Read the model definition and answer for the solid it produces. Units are mm, in the model's axes. Face numbers are marked on the shaded views. A direction names the side the tool comes from. Round coordinates to 2 decimals unless told otherwise and drop trailing zeros. Order: outer loops, then holes, each group sorted by start corner. A loop starts at its lowest first (then second) coordinate and runs counter-clockwise, first axis right, second up. Notation, with made-up numbers: (88, 85) - (140, 85) arc R21 cw to (140, 97) - close; hole circle Ø8 at (25.25, 75). An arc over 180 degrees is marked (long way). Answer as a JSON object with one key per item and string values. Group by question number.
Q1. A tool of negligible diameter and unlimited length cuts with its end or side. For the marked faces 1, 2 and 3, from which of +Z, -Z, +X, -X, +Y, -Y can it reach the whole face along a straight path? Write none if from no direction.
Q2. The mould has two halves that part along Y. Classify the marked faces 4, 5 and 6: pulls with the +Y half, pulls with the -Y half, needs draft (parallel to the pull), parting line crosses it, or undercut.
Q3. A cutting plane is placed at B-B on x = -11.5. Determine the outline of the cut face in (y, z).
Q4. Given pin 1 Ø2 at (x, y) = (14.5, -5) entering from -Z; pin 2 Ø3 at (x, y) = (7, -3) entering from -Z; pin 3 Ø0.7 at (x, y) = (-13.5, -5) entering from -Z; pin 4 Ø1 at (y, z) = (9, 1) entering from +X, each flat-ended and moving along its own axis, determine where each tip first touches the part or whether it passes through.
Q5. A cutting plane is placed at A-A on y = 0. Determine the outline of the cut face in (x, z).
Q6. Consider line 1 (Y direction, x = -13, z = 1.25) (3 decimals); line 2 (Y direction, x = 10.5, z = 1); line 3 (Y direction, x = -14, z = 4). Determine where each line is inside the solid, lowest interval first.
```python
from build123d import *

# Parameters (mm, degrees)
BOSS_EXTRUDE1_DEPTH     = 2
SKETCH2_R               = 1.54
BOSS_EXTRUDE2_DEPTH     = 4
SKETCH3_R               = 3.5
BOSS_EXTRUDE3_DEPTH     = 1
SKETCH4_W               = 2
SKETCH4_H               = 17
BOSS_EXTRUDE4_DEPTH     = 0.001
SKETCH5_W               = 18
SKETCH5_H               = 2
BOSS_EXTRUDE5_DEPTH     = 0.001
SKETCH6_W               = 2.001
SKETCH6_H               = 2
BOSS_EXTRUDE6_DEPTH     = 5
BOSS_EXTRUDE7_DEPTH     = 0.001
CUT_EXTRUDE1_DEPTH      = 20.519323784
SKETCH9_W               = 2.937742252
SKETCH9_H               = 8
CUT_EXTRUDE2_DEPTH      = 0.001
CUT_EXTRUDE11_START     = -0.001
SKETCH21_R              = 9.75
SKETCH21_R_2            = 3.5
CUT_EXTRUDE11_DEPTH     = 0.001
SKETCH10_W              = 32
SKETCH10_H              = 2
BOSS_EXTRUDE8_DEPTH     = 7
FILLET1_R               = 0.5
SKETCH11_R              = 0.625
BOSS_EXTRUDE9_DEPTH     = 2
SKETCH14_W              = 2
SKETCH14_H              = 2
CUT_EXTRUDE5_DEPTH      = 22.401355237
SKETCH12_R              = 0.675
CUT_EXTRUDE3_DEPTH      = 2.5
CUT_EXTRUDE6_DEPTH      = 2
FILLET2_R               = 0.5
FILLET3_R               = 0.5
FILLET4_R               = 2
CUT_EXTRUDE7_DEPTH      = 26.019992106
CUT_EXTRUDE7_DEPTH_BACK = 1
SKETCH19_R              = 0.625
CUT_EXTRUDE9_DEPTH      = 2


with BuildPart() as part:
    # Sketch1 → Boss-Extrude1 (new body)
    with BuildSketch(Plane.XY):
        Polygon((-11, 6), (-11, 11), (11, 11), (11, 6), (11, -6), (-11, -6), align=None)
    extrude(amount=BOSS_EXTRUDE1_DEPTH)

    # Sketch3 → Boss-Extrude3 (add)
    with BuildSketch(Plane(origin=(0, 0, 0), x_dir=(-1, 0, 0), z_dir=(0, 0, -1))):
        with Locations(Location((0, 0, 0), (0, 0, 180))):
            Circle(SKETCH3_R)
    extrude(amount=BOSS_EXTRUDE3_DEPTH)

    # Sketch4 → Boss-Extrude4 (add)
    with BuildSketch(Plane(origin=(0, 0, 0), x_dir=(-1, 0, 0), z_dir=(0, 0, -1))):
        with Locations((10, 2.5)):
            Rectangle(SKETCH4_W, SKETCH4_H)
        with Locations((-10, 2.5)):
            Rectangle(SKETCH4_W, SKETCH4_H)
    extrude(amount=BOSS_EXTRUDE4_DEPTH)

    # Sketch5 → Boss-Extrude5 (add)
    with BuildSketch(Plane(origin=(0, 0, 0), x_dir=(-1, 0, 0), z_dir=(0, 0, -1))):
        with Locations((0, 10)):
            Rectangle(SKETCH5_W, SKETCH5_H)
    extrude(amount=BOSS_EXTRUDE5_DEPTH)

    # Sketch6 → Boss-Extrude6 (add)
    with BuildSketch(Plane(origin=(11, 0, 0), x_dir=(0, 0, -1), z_dir=(1, 0, 0))):
        with Locations((-0.9995, -5)):
            Rectangle(SKETCH6_W, SKETCH6_H)
        with Locations((-0.9995, 5)):
            Rectangle(SKETCH6_W, SKETCH6_H)
    boss_extrude6 = extrude(amount=BOSS_EXTRUDE6_DEPTH)

    # Mirror1: Boss-Extrude6 across plane
    add(boss_extrude6.mirror(Plane(origin=(0, 0, 0), x_dir=(0, 0, 1), z_dir=(1, 0, 0))))

    # Sketch7 → Boss-Extrude7 (add)
    with BuildSketch(Plane(origin=(0, 0, -0.001), x_dir=(-1, 0, 0), z_dir=(0, 0, -1))):
        with BuildLine():
            ThreePointArc((-6.708203932, -6), (-8.407551231, -3.211398808), (-9, 0))
            Line((-9, 0), (-9, -6))
            Line((-9, -6), (-6.708203932, -6))
        make_face()
        with BuildLine():
            Line((-9, 9), (-9, 0))
            ThreePointArc((-9, 0), (-6.363961031, 6.363961031), (0, 9))
            Line((0, 9), (-9, 9))
        make_face()
    boss_extrude7 = extrude(amount=-BOSS_EXTRUDE7_DEPTH)

    # Sketch8 → Cut-Extrude1 (cut, through all)
    with BuildSketch(Plane(origin=(0, 0, -0.001), x_dir=(-1, 0, 0), z_dir=(0, 0, -1))):
        with BuildLine():
            Line((-11, 4), (-9.16515139, 4))
            ThreePointArc((-9.16515139, 4), (-10, 0), (-9.16515139, -4))
            Line((-9.16515139, -4), (-11, -4))
            Line((-11, -4), (-11, 4))
        make_face()
    cut_extrude1 = extrude(amount=-CUT_EXTRUDE1_DEPTH, mode=Mode.SUBTRACT)

    # Sketch9 → Cut-Extrude2 (cut)
    with BuildSketch(Plane(origin=(0, 0, -0.001), x_dir=(-1, 0, 0), z_dir=(0, 0, -1))):
        with Locations((-9.531128874, 0)):
            Rectangle(SKETCH9_W, SKETCH9_H)
    cut_extrude2 = extrude(amount=-CUT_EXTRUDE2_DEPTH, mode=Mode.SUBTRACT)

    # Mirror2: Boss-Extrude7, Cut-Extrude1, Cut-Extrude2 across plane
    add(boss_extrude7.mirror(Plane(origin=(0, 0, 0), x_dir=(0, 0, 1), z_dir=(1, 0, 0))))
    add(cut_extrude1.mirror(Plane(origin=(0, 0, 0), x_dir=(0, 0, 1), z_dir=(1, 0, 0))), mode=Mode.SUBTRACT)
    add(cut_extrude2.mirror(Plane(origin=(0, 0, 0), x_dir=(0, 0, 1), z_dir=(1, 0, 0))), mode=Mode.SUBTRACT)

    # Sketch21 → Cut-Extrude11 (cut)
    with BuildSketch(Plane(origin=(0, 0, -0.001), x_dir=(-1, 0, 0), z_dir=(0, 0, -1)).offset(CUT_EXTRUDE11_START)):
        Circle(SKETCH21_R)
        with Locations(Location((0, 0, 0), (0, 0, 180))):
            Circle(SKETCH21_R_2, mode=Mode.SUBTRACT)
    extrude(amount=CUT_EXTRUDE11_DEPTH, mode=Mode.SUBTRACT)

    # Sketch10 → Boss-Extrude8 (add)
    with BuildSketch(Plane.XY.offset(2)):
        with Locations((0, -5)):
            Rectangle(SKETCH10_W, SKETCH10_H)
        with Locations((0, 5)):
            Rectangle(SKETCH10_W, SKETCH10_H)
    extrude(amount=BOSS_EXTRUDE8_DEPTH)

    # Fillet1
    fillet1_edges = [part.edges().sort_by_distance(p)[0] for p in [
        (10, 0, 2),
        (-10, 0, 2),
    ]]
    fillet(fillet1_edges, radius=FILLET1_R)

    # Sketch11 → Boss-Extrude9 (add)
    with BuildSketch(Plane(origin=(0, 0, -0.001), x_dir=(-1, 0, 0), z_dir=(0, 0, -1))):
        with Locations(Location((-13, -5, 0), (0, 0, 180))):
            Circle(SKETCH11_R)
    boss_extrude9 = extrude(amount=BOSS_EXTRUDE9_DEPTH)

    # Sketch14 → Cut-Extrude5 (cut, through all)
    with BuildSketch(Plane(origin=(0, 0, -0.001), x_dir=(-1, 0, 0), z_dir=(0, 0, -1))):
        with Locations((10, 7)):
            Rectangle(SKETCH14_W, SKETCH14_H)
        with Locations((-10, 7)):
            Rectangle(SKETCH14_W, SKETCH14_H)
    extrude(amount=-CUT_EXTRUDE5_DEPTH, mode=Mode.SUBTRACT)

    # Sketch12 → Cut-Extrude3 (cut)
    with BuildSketch(Plane(origin=(0, 0, -0.001), x_dir=(-1, 0, 0), z_dir=(0, 0, -1))):
        with Locations((13, -5)):
            Circle(SKETCH12_R)
    cut_extrude3 = extrude(amount=-CUT_EXTRUDE3_DEPTH, mode=Mode.SUBTRACT)

    # Sketch16 → Cut-Extrude6 (cut)
    with BuildSketch(Plane(origin=(0, 6, 0), x_dir=(1, 0, 0), z_dir=(0, 1, 0))):
        with BuildLine():
            Line((-9, -1), (-9, -2))
            ThreePointArc((-9, -2), (-8.75, -1.5), (-9, -1))
        make_face()
    cut_extrude6 = extrude(amount=CUT_EXTRUDE6_DEPTH, mode=Mode.SUBTRACT)

    # Mirror3: Boss-Extrude9, Cut-Extrude3 across plane
    add(boss_extrude9.mirror(Plane.ZX))
    add(cut_extrude3.mirror(Plane.ZX), mode=Mode.SUBTRACT)

    # Mirror4: Cut-Extrude6 across plane
    add(cut_extrude6.mirror(Plane(origin=(0, 0, 0), x_dir=(0, 0, 1), z_dir=(1, 0, 0))), mode=Mode.SUBTRACT)

    # Fillet2
    fillet2_edges = [part.edges().sort_by_distance(p)[0] for p in [
        (12.375, -5, -0.001),
        (12.375, 5, -0.001),
    ]]
    fillet(fillet2_edges, radius=FILLET2_R)

    # Fillet3
    # the kernel refuses this fillet: 0.5 mm, written as the material it takes off along each edge
    with BuildSketch(Plane(origin=(-13, -5, -0.001), x_dir=(-1, 0, 0), z_dir=(0, -1, 0))) as fillet3_piece_1:
        with BuildLine():
            CenterArc((0.675 + FILLET3_R, -FILLET3_R), FILLET3_R, 90, 90)
            Line((0.675, -FILLET3_R), (0.675, 0))
            Line((0.675, 0), (0.675 + FILLET3_R, 0))
        make_face()
    revolve(axis=Axis((-13, -5, -0.001), (0, 0, -1)), mode=Mode.SUBTRACT)
    with BuildSketch(Plane(origin=(-13, 5, -0.001), x_dir=(-1, 0, 0), z_dir=(0, 1, 0))) as fillet3_piece_2:
        with BuildLine():
            CenterArc((0.675 + FILLET3_R, FILLET3_R), FILLET3_R, 180, 90)
            Line((0.675, FILLET3_R), (0.675, 0))
            Line((0.675, 0), (0.675 + FILLET3_R, 0))
        make_face()
    revolve(axis=Axis((-13, 5, -0.001), (0, 0, 1)), mode=Mode.SUBTRACT)

    # Fillet4
    fillet4_edges = [part.edges().sort_by_distance(p)[0] for p in [
        (16, -5, 9),
        (-16, -5, 9),
        (-16, 5, 9),
        (16, 5, 9),
    ]]
    fillet(fillet4_edges, radius=FILLET4_R)

    # Sketch17 → Cut-Extrude7 (cut, two sides: drawn at the far end of the back side and taken through both)
    with BuildSketch(Plane.XZ.offset(6).offset(-CUT_EXTRUDE7_DEPTH_BACK)):
        with BuildLine():
            Line((-16, 7), (-16, -0.001))
            Line((-16, -0.001), (-14.5, -0.001))
            Line((-14.5, -0.001), (-14.5, 7))
            ThreePointArc((-14.5, 7), (-14.353553391, 7.353553391), (-14, 7.5))
            Line((-14, 7.5), (14, 7.5))
            ThreePointArc((14, 7.5), (14.353553391, 7.353553391), (14.5, 7))
            Line((14.5, 7), (14.5, -0.001))
            Line((14.5, -0.001), (16, -0.001))
            Line((16, -0.001), (16, 7))
            ThreePointArc((16, 7), (15.414213562, 8.414213562), (14, 9))
            Line((14, 9), (-14, 9))
            ThreePointArc((-14, 9), (-15.414213562, 8.414213562), (-16, 7))
        make_face()
    extrude(amount=CUT_EXTRUDE7_DEPTH + CUT_EXTRUDE7_DEPTH_BACK, mode=Mode.SUBTRACT)

    # Sketch19 → Cut-Extrude9 (cut)
    with BuildSketch(Plane(origin=(0, 6, 0), x_dir=(1, 0, 0), z_dir=(0, 1, 0))):
        with Locations(Location((0, -2.625, 0), (0, 0, 90))):
            Circle(SKETCH19_R)
        with Locations(Location((0, -8.125, 0), (0, 0, 270))):
            Circle(SKETCH19_R)
    extrude(amount=-CUT_EXTRUDE9_DEPTH, mode=Mode.SUBTRACT)


with BuildPart() as body_2:
    # Sketch2 → Boss-Extrude2 (new body)
    with BuildSketch(Plane(origin=(0, 0, 2), x_dir=(-1, 0, 0), z_dir=(0, 0, -1))):
        Circle(SKETCH2_R)
    extrude(amount=BOSS_EXTRUDE2_DEPTH)


with BuildPart() as part_1:
    add(part.part)

    # Combine2: cut body 2
    add(body_2.part, mode=Mode.SUBTRACT)


solid = part_1.part
```
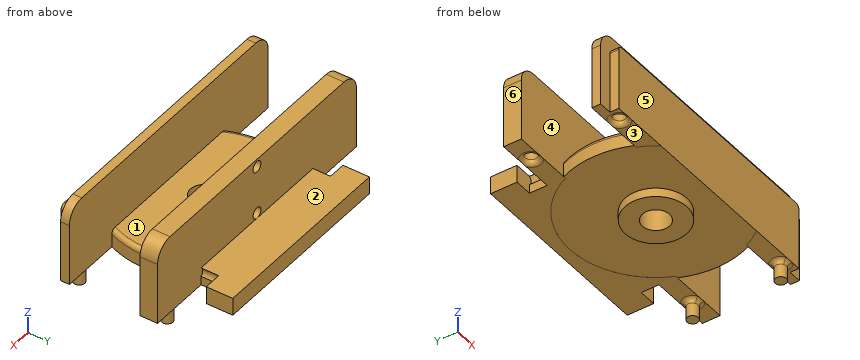
Result set:
{
 "1": {"face 1": "+Z, +X, -X", "face 2": "+Z, +X, -X, +Y", "face 3": "-Z, -X, +Y, -Y"},
 "2": {"face 4": "undercut", "face 5": "pulls with the -Y half", "face 6": "needs draft"},
 "3": {"outline": "(-6, 0) - (-4, 0) - (-4, 9) - (-5, 9) - (-5, 7.5) - (-6, 7.5) - close; (4, 0) - (6, 0) - (6, 9) - (4, 9) - close"},
 "4": {"pin 1": "stops at z = -2", "pin 2": "stops at z = 0", "pin 3": "stops at z = 0.12", "pin 4": "stops at x = 11"},
 "5": {"outline": "(-10, 0) - (-3.5, 0) - (-3.5, -1) - (-1.54, -1) - (-1.54, 2) - (-9.5, 2) arc R0.5 ccw to (-10, 1.5) - close; (1.54, -1) - (3.5, -1) - (3.5, 0) - (10, 0) - (10, 1.5) arc R0.5 ccw to (9.5, 2) - (1.54, 2) - close"},
 "6": {"line 1": "y = -6 to -5.675, -4.325 to -4, 4 to 4.325, 5.675 to 6", "line 2": "y = -6 to -4, 4 to 6, 8 to 11", "line 3": "y = -6 to -4, 4 to 6"}
}
